Can you work these out from the model? Positions are in its coordinate system, mm. A direction names the side the tool comes from. Coordinates: 2 decimals unless noted, no trailing zeros. Order: outer loops, then holes, each group sorted by start corner. A loop starts at its lowest first (then second) coordinate and runs counter-clockwise, first axis right, second up. Notation, with made-up numbers: (-5, 52) -> (39, 52) arc R30 ccw to (39, 87) -> close; hole circle Ø10 at (67.25, 0.5). An arc over 180 degrees is marked (long way). Return JSON: item names as keys, results as strings. Group by question number.
1) If we section it at C-C, the plane x = -66.5: Please give me the cut outline in (y, z), then the cut area to 3 significant figures.
2) If we section it at D-D, the plane y = -21.5: Please give me the cut outline in (x, z), then the cut area to 3 significant figures.
3) If we section it at B-B, the plane y = -74: Please give me the cut outline in (x, z), then the cut area to 3 significant figures.
4) If we section it at A-A, the plane z = 10.5: Please give me the cut outline in (x, y).
5) If I drill on probe 1 along X at (y, z) = (-8.5, -17); probe 2 along Y at (x, z) = (-14.5, 13.5); probe 3 along Y at (x, z) = (59.5, -13.5), over which ranges is the centre line in solid material (lowest first)? Write a range as from..to.
6) For faces 5 (the flat face through (-115.937, -72.421, 0.284)), 6 (the flat face through (-64.09, -75.024, -0.284)), which set-ups out of +Z, -Z, +X, -X, +Y, -Y let a thin tool reach every point of the face, with its end or its side?
7) Thinking about a two-plate mould opening in X: for faces 1 (the flat face through (63.966, 59.236, -0.284)), 2 (the flat face through (82, 81.852, 0)), 3 (the cylindrical face through (68.856, -49.862, 0.284)), 4 (the flat face through (97.714, -9, 0)), which applies, +X half, -X half, draft (parallel to the pull), parting line (faces both ways), or undercut?
8) For pin 1 (2 mm diameter, centred on x = -41.97, y = -91.36, fed in from +Z); pin 2 (10 mm diameter, centred on y = -18, z = -15, fed in from -X); pin 3 (3 mm diameter, centred on x = 91.36, y = -91.36, fed in from -Z), each with a flat end and sliding along its axis, tell me the tip position at first contact or that it passes through.
from build123d import *

# Parameters (mm, degrees)
BOSS_EXTRUDE1_DEPTH = 40.64
SKETCH6_R           = 1.1303
CUT_EXTRUDE1_DEPTH  = 158.779215984
SKETCH7_R           = 19.05
CUT_EXTRUDE2_DEPTH  = 158.779215984


with BuildPart() as part:
    # Sweep3: sweep along a path in Sketch2
    with BuildLine(Plane.XY) as sweep3_path:
        Line((-111.378641457, -46.568583299), (-11.322173751, -64.21123815))
        ThreePointArc((-11.322173751, -64.21123815), (53.410187761, -37.398216088), (56.466415172, 32.6009))
        Line((56.466415172, 32.6009), (37.416415172, 65.596467884))
    # 3DSketch1 → Sweep3 (sweep)
    with BuildSketch(Plane(origin=(-117.024291009, -78.586652965, -20.32), x_dir=(0.051794909001673446, 0.2937435257699459, 0.9544799780350292), z_dir=(0.984807753012208, -0.17364817766693055, 0))):
        Polygon((0, 0), (3.788092413, -12.121895721), (42.57815872, 0), (38.790066307, 12.121895721), align=None)
    sweep(path=sweep3_path.line)

    # Sketch5 → Boss-Extrude1 (add)
    with BuildSketch(Plane.XY.offset(20.32)):
        with BuildLine():
            Line((-16.967823303, -96.229307816), (-117.024291009, -78.586652965))
            Line((-117.024291009, -78.586652965), (-117.024291009, -97.7138))
            Line((-117.024291009, -97.7138), (3.02e-07, -97.7138))
            ThreePointArc((3.02e-07, -97.7138), (-8.516318665, -97.341969504), (-16.967823303, -96.229307816))
        make_face()
        with BuildLine():
            ThreePointArc((97.7138, -9e-08), (69.09409067, -69.094090521), (3.02e-07, -97.7138))
            Line((3.02e-07, -97.7138), (97.7138, -97.7138))
            Line((97.7138, -97.7138), (97.7138, -9e-08))
        make_face()
        with BuildLine():
            ThreePointArc((84.6226331, 48.8569), (94.384283017, 25.290192366), (97.7138, -9e-08))
            Line((97.7138, -9e-08), (97.7138, 81.852467884))
            Line((97.7138, 81.852467884), (65.5726331, 81.852467884))
            Line((65.5726331, 81.852467884), (84.6226331, 48.8569))
        make_face()
    extrude(amount=-BOSS_EXTRUDE1_DEPTH)

    # Sketch6 → Cut-Extrude1 (cut, through all)
    with BuildSketch(Plane.XY.offset(20.32)):
        with Locations((91.3638, -91.3638)):
            Circle(SKETCH6_R)
        with Locations((-41.9735, -91.3638)):
            Circle(SKETCH6_R)
    extrude(amount=-CUT_EXTRUDE1_DEPTH, mode=Mode.SUBTRACT)

    # Sketch7 → Cut-Extrude2 (cut, through all)
    with BuildSketch(Plane.XY.offset(20.32)):
        with Locations((-117.024291009, -97.7138)):
            Circle(SKETCH7_R)
    extrude(amount=-CUT_EXTRUDE2_DEPTH, mode=Mode.SUBTRACT)


solid = part.part
Result sheet:
{
 "1": {"outline": "(-97.71, -20.32) -> (-74.6, -20.32) -> (-74.6, 20.32) -> (-97.71, 20.32) -> close", "area": "939 mm2"},
 "2": {"outline": "(82.25, -20.32) -> (97.71, -20.32) -> (97.71, 20.32) -> (82.25, 20.32) -> close", "area": "628 mm2"},
 "3": {"outline": "(-116.22, -20.32) -> (-69.9, -20.32) -> (-69.9, 20.32) -> (-116.22, 20.32) -> close; (41.85, -20.32) -> (97.71, -20.32) -> (97.71, 20.32) -> (41.85, 20.32) -> close", "area": "4,150 mm2"},
 "4": {"outline": "(-117.02, -78.66) arc R19.05 cw to (-97.97, -97.71) -> (97.71, -97.71) -> (97.71, 81.85) -> (65.57, 81.85) -> (54.57, 75.5) -> (73.62, 42.51) arc R85.01 cw to (-14.76, -83.72) -> (-114.82, -66.08) -> (-117.02, -78.59) -> close; hole circle Ø2.26 at (-41.97, -91.36); hole circle Ø2.26 at (91.36, -91.36)"},
 "5": {"probe 1": "x = 84.59..97.71", "probe 2": "y = -97.71..-83.77", "probe 3": "y = -97.71..-60.72, 66.97..78.35"},
 "6": {"face 5": "+Z, -Z, -X, +Y", "face 6": "+Z, -Z, +Y"},
 "7": {"face 1": "-X half", "face 2": "draft", "face 3": "undercut", "face 4": "+X half"},
 "8": {"pin 1": "passes through", "pin 2": "stops at x = 81.84", "pin 3": "stops at z = -20.32"}
}
